Read the model definition and answer for the solid it produces. Units are mm, in the model's axes. A direction names the side the tool comes from. Give positions to 0.01 mm unless a question says otherwise; leave off trailing zeros. Loops run counter-clockwise (first coordinate to the right, second up) from the corner with the lowest first, then second, coordinate; pieces in that order, holes last.
(1) Find section A-A, the plane z = 46. Write down the section's boundary in (x, y), then the cut area to 3 significant figures.
(2) Which of the six approach directions +Z, -Z, +X, -X, +Y, -Y give full straight-line access (tool end or side, diameter ignored) to faces 1 (the face through (22, 1.5, 64)), 2 (the face through (13, 16, 46))?
(3) Determine the mould class of faces 3 (the face through (25, 21, 23)), 4 (the face through (40, 16, 44)), 5 (the face through (-30, 16, 32)) for opening direction Z: pulls with the +Z half, pulls with the -Z half, needs draft (parallel to the pull), parting line crosses it, or undercut.
(4) Find section B-B, the plane x = 5. Write down the section's boundary in (y, z), then the cut area to 3 significant figures.
(5) Each of these flat-tipped pins is pushed along its axis until it touches: P1, Ø5.5, axis at y = 18.5, z = 5.5, coming from the -X side; P2, Ø12, axis at x = 12.5, z = 25.5, coming from the +Y side; P3, Ø5, axis at y = 27.5, z = 8.5, coming from the +X side. Where does it stop, or does it pass through?
(6) Find section C-C, the plane z = 24.5. Write down the section's boundary in (x, y), then the cut area to 3 significant figures.
(7) Straight lines are drawn through the part: probe 1 along Y at (x, z) = (45, 1); probe 2 along X at (y, z) = (27, 1); probe 3 along X at (y, z) = (16, 24.5). For each, find the intervals that lie inside material, in ascending order.
(8) Find section D-D, the plane y = 18.5. Write down the section's boundary in (x, z), then the cut area to 3 significant figures.
```python
from build123d import *

# Parameters (mm, degrees)
PAD005_DEPTH  = 50
PAD006_DEPTH  = 50
SKETCH013_R   = 6.6
PAD011_DEPTH  = 30
SKETCH014_R   = 6.6
PAD012_DEPTH  = 35
SKETCH009_W   = 11
SKETCH009_H   = 10
PAD007_DEPTH  = 14
SKETCH010_W   = 11
SKETCH010_H   = 10
PAD008_DEPTH  = 14
SKETCH011_W   = 11
SKETCH011_H   = 10
PAD009_DEPTH  = 14
SKETCH012_W   = 11
SKETCH012_H   = 10
PAD010_DEPTH  = 14
SKETCH001_W   = 32
SKETCH001_H   = 4
PAD001_DEPTH  = 50
SKETCH004_R   = 2.75
HOLE_DEPTH    = 4.001
PAD003_DEPTH  = 20
SKETCH002_W   = 37
SKETCH002_H   = 18
PAD002_DEPTH  = 35
SKETCH005_W   = 16
SKETCH005_H   = 30
PAD004_DEPTH  = 30
SKETCH006_R   = 6.6
HOLE001_DEPTH = 30.001
SKETCH_W      = 32
SKETCH_H      = 41
PAD_DEPTH     = 50


with BuildPart() as body005:
    # Sketch007 (on Face1 of CopyPad004) → Pad005 (new body)
    with BuildSketch(Plane(origin=(0, 0, 0), x_dir=(0, -1, 0), z_dir=(-1, 0, 0))):
        Polygon((0, 3), (-11, 13.048009), (-11, 44), (0, 44), align=None)
    extrude(amount=-PAD005_DEPTH)


with BuildPart() as body006:
    # Sketch008 (on Face1 of CopyPad005) → Pad006 (new body)
    with BuildSketch(Plane(origin=(0, 0, 0), x_dir=(0, -1, 0), z_dir=(-1, 0, 0))):
        Polygon((-32, 44), (-21, 44), (-21, 12.966247), (-32, 3), align=None)
    extrude(amount=-PAD006_DEPTH)


with BuildPart() as body011:
    # Sketch013 (on Face1 of CopyPad006001) → Pad011 (new body)
    with BuildSketch(Plane(origin=(0, 32, 0), x_dir=(-1, 0, 0), z_dir=(0, 1, 0))):
        with Locations((-37, 28)):
            Circle(SKETCH013_R)
    extrude(amount=-PAD011_DEPTH)


with BuildPart() as body012:
    # Sketch014 (on Face1 of CopyPad006002) → Pad012 (new body)
    with BuildSketch(Plane(origin=(0, 32, 0), x_dir=(-1, 0, 0), z_dir=(0, 1, 0))):
        with Locations((-13, 28)):
            Circle(SKETCH014_R)
    extrude(amount=-PAD012_DEPTH)


with BuildPart() as body007:
    # Sketch009 (on Face1 of CopyPad006) → Pad007 (new body)
    with BuildSketch(Plane.YZ.offset(50)):
        with Locations((26.5, 8)):
            Rectangle(SKETCH009_W, SKETCH009_H)
    extrude(amount=-PAD007_DEPTH)


with BuildPart() as body008:
    # Sketch010 (on Face1 of CopyPad005001) → Pad008 (new body)
    with BuildSketch(Plane.YZ.offset(50)):
        with Locations((5.5, 8)):
            Rectangle(SKETCH010_W, SKETCH010_H)
    extrude(amount=-PAD008_DEPTH)


with BuildPart() as body009:
    # Sketch011 (on Face1 of CopyPad005002) → Pad009 (new body)
    with BuildSketch(Plane(origin=(0, 0, 0), x_dir=(0, -1, 0), z_dir=(-1, 0, 0))):
        with Locations((-5.5, 8)):
            Rectangle(SKETCH011_W, SKETCH011_H)
    extrude(amount=-PAD009_DEPTH)


with BuildPart() as body010:
    # Sketch012 (on Face1 of CopyPad005003) → Pad010 (new body)
    with BuildSketch(Plane(origin=(0, 0, 0), x_dir=(0, -1, 0), z_dir=(-1, 0, 0))):
        with Locations((-26.5, 8)):
            Rectangle(SKETCH012_W, SKETCH012_H)
    extrude(amount=-PAD010_DEPTH)


with BuildPart() as body001:
    # Sketch001 (on Face1 of CopyPad) → Pad001 (new body)
    with BuildSketch(Plane.YZ.offset(50)):
        with Locations((16, 1)):
            Rectangle(SKETCH001_W, SKETCH001_H)
    extrude(amount=-PAD001_DEPTH)

    # Sketch004 (on Face3 of Pad001) → Hole (cut, through all)
    with BuildSketch(Plane(origin=(50, 0, -1), x_dir=(1, 0, 0), z_dir=(0, 0, -1))):
        with Locations((-45, -5)):
            Circle(SKETCH004_R)
        with Locations((-5, -5)):
            Circle(SKETCH004_R)
        with Locations((-5, -27)):
            Circle(SKETCH004_R)
        with Locations((-45, -27)):
            Circle(SKETCH004_R)
    extrude(amount=-HOLE_DEPTH, mode=Mode.SUBTRACT)


with BuildPart() as body003:
    # Sketch003 (on Face1 of CopyPad002) → Pad003 (new body)
    with BuildSketch(Plane.YZ.offset(31)):
        Polygon((9.5, 79.211134), (22.5, 79.211134), (22.5, 74.211134), (30.5, 74.211134), (30.5, 53.183285), (25.112084, 49.00605), (6.112084, 49.00605), (1.5, 53.183285), (1.5, 74.211134), (9.5, 74.211134), align=None)
    extrude(amount=-PAD003_DEPTH)


with BuildPart() as body002:
    # Sketch002 (on Face1 of CopyPad001) → Pad002 (new body)
    with BuildSketch(Plane(origin=(0, 0, 44), x_dir=(0, -1, 0), z_dir=(0, 0, 1))):
        with Locations((-15.5, 22)):
            Rectangle(SKETCH002_W, SKETCH002_H)
    extrude(amount=PAD002_DEPTH)

    # Boolean: cut Body003
    add(body003.part, mode=Mode.SUBTRACT)


with BuildPart() as body004:
    # Sketch005 (on Face1 of CopyPad003) → Pad004 (new body)
    with BuildSketch(Plane(origin=(0, 0, 0), x_dir=(0, -1, 0), z_dir=(-1, 0, 0))):
        with Locations((-16, 32)):
            Rectangle(SKETCH005_W, SKETCH005_H)
    extrude(amount=PAD004_DEPTH)

    # Sketch006 (on Face3 of Pad004) → Hole001 (cut, through all)
    with BuildSketch(Plane(origin=(0, 0, 17), x_dir=(1, 0, 0), z_dir=(0, 0, -1))):
        with Locations((-21, -16)):
            Circle(SKETCH006_R)
    extrude(amount=-HOLE001_DEPTH, mode=Mode.SUBTRACT)


with BuildPart() as body:
    # Sketch → Pad (new body)
    with BuildSketch(Plane.YZ):
        with Locations((16, 23.5)):
            Rectangle(SKETCH_W, SKETCH_H)
    extrude(amount=PAD_DEPTH)

    # Boolean001: cut Body005
    add(body005.part, mode=Mode.SUBTRACT)

    # Boolean002: cut Body006
    add(body006.part, mode=Mode.SUBTRACT)

    # Boolean003: cut Body011
    add(body011.part, mode=Mode.SUBTRACT)

    # Boolean004: cut Body012
    add(body012.part, mode=Mode.SUBTRACT)

    # Boolean005: cut Body007
    add(body007.part, mode=Mode.SUBTRACT)

    # Boolean006: cut Body008
    add(body008.part, mode=Mode.SUBTRACT)

    # Boolean007: cut Body009
    add(body009.part, mode=Mode.SUBTRACT)

    # Boolean008: cut Body010
    add(body010.part, mode=Mode.SUBTRACT)

    # Boolean009: union Body001
    add(body001.part)

    # Boolean010: union Body002
    add(body002.part)

    # Boolean011: union Body004
    add(body004.part)


solid = body.part
```
Entries:
1. outline: (-30, 8) - (0, 8) - (0, 24) - (-30, 24) - close; (13, -3) - (31, -3) - (31, 34) - (13, 34) - close; hole circle Ø13.2 at (-21, 16)
1. area: 1,010 mm2
2. face 1: +X, -X
2. face 2: +Z, +Y, -Y
3. face 3: undercut
3. face 4: pulls with the +Z half
3. face 5: needs draft
4. outline: (0, -1) - (2.25, -1) - (2.25, 3) - (0, 3) - close; (7.75, -1) - (24.25, -1) - (24.25, 3) - (21, 3) - (21, 44) - (11, 44) - (11, 13.05) - (10.95, 13) - (11, 13) - (11, 3) - (7.75, 3) - close; (29.75, -1) - (32, -1) - (32, 3) - (29.75, 3) - close
4. area: 494 mm2
5. P1: stops at x = 0
5. P2: stops at y = 21
5. P3: stops at x = 36
6. outline: (-30, 8) - (0, 8) - (0, 11) - (7.4, 11) - (7.4, 21) - (0, 21) - (0, 24) - (-30, 24) - close; (18.6, 11) - (31.4, 11) - (31.4, 21) - (18.6, 21) - close; (42.6, 11) - (50, 11) - (50, 21) - (42.6, 21) - close; hole circle Ø13.2 at (-21, 16)
6. area: 619 mm2
7. probe 1: y = 0 to 2.25, 7.75 to 24.25, 29.75 to 32
7. probe 2: x = 0 to 2.25, 7.75 to 42.25, 47.75 to 50
7. probe 3: x = -30 to -27.6, -14.4 to 7.4, 18.6 to 31.4, 42.6 to 50
8. outline: (-30, 17) - (-27.11, 17) - (-27.11, 47) - (-30, 47) - close; (-14.89, 17) - (0, 17) - (0, -1) - (50, -1) - (50, 44) - (31, 44) - (31, 49.01) - (13, 49.01) - (13, 44) - (0, 44) - (0, 47) - (-14.89, 47) - close; hole circle Ø13.2 at (13, 28); hole circle Ø13.2 at (37, 28)
8. area: 2,600 mm2
